Input: part model. Units: mm. Frame: model coordinates. A direction names the side the tool comes from. Give positions to 0.01 mm unless a question says otherwise; leave off trailing zeros. Loops run counter-clockwise (first coordinate to the right, second up) from the corner with the lowest first, then second, coordinate; pieces in that order, holes last. Notation, with made-up numbers: (-31, -10.5) - (-18, -10.5) arc R18 cw to (-18, 7.5) - close; hole circle Ø3 at (72, 38.25). An arc over 180 degrees is marked (long way). Answer as a JSON object with one key per item and string values.
from build123d import *

# Parameters (mm, degrees)
BOSS_EXTRUDE1_DEPTH  = 45.4
LPATTERN1_COUNT      = 2
LPATTERN1_PITCH      = 20
LPATTERN1_COUNT_DIR2 = 2
LPATTERN1_PITCH_DIR2 = 20


with BuildPart() as part:
    # Sketch1 → Boss-Extrude1 (new body)
    with BuildSketch(Plane(origin=(0, 0, 0), x_dir=(0, 0, -1), z_dir=(1, 0, 0))):
        Polygon((19.5, 5.941454138), (19.5, 0), (27, 0), (27, 13), (0, 13), (0, 0), (7.5, 0), (7.5, 5.941454138), align=None)
        with BuildLine():
            Line((7.5, 3.45), (7.5, 2.55))
            ThreePointArc((7.5, 2.55), (7.95, 3), (7.5, 3.45))
        make_face()
        with BuildLine():
            ThreePointArc((19.5, 3.45), (19.05, 3), (19.5, 2.55))
            Line((19.5, 2.55), (19.5, 3.45))
        make_face()
    extrude(amount=BOSS_EXTRUDE1_DEPTH)

    # Sketch3 → M3x0.5 Tapped Hole1 (revolve, cut)
    with BuildSketch(Plane(origin=(12.7, 13, -23.5), x_dir=(0, 0, 1), z_dir=(1, 0, 0))):
        Polygon((0, 0), (0, 4.251075774), (1.25, 3.5), (1.25, 0), align=None)
    m3x0_5_tapped_hole1 = revolve(axis=Axis((12.7, 19.35, -23.5), (0, -1, 0)), mode=Mode.SUBTRACT)

    # LPattern1: M3x0.5 Tapped Hole1 2 × 2
    with Locations(*[(i * LPATTERN1_PITCH, 0, j * LPATTERN1_PITCH_DIR2) for i in range(LPATTERN1_COUNT) for j in range(LPATTERN1_COUNT_DIR2) if (i, j) != (0, 0)]):
        add(m3x0_5_tapped_hole1, mode=Mode.SUBTRACT)


solid = part.part
Item 1: Cut plane B-B (x = 28.5). Return loops of the section in (y, z), then the cut area to 3 significant figures.
Geometry check:
{"outline": "(0, -27) - (13, -27) - (13, 0) - (0, 0) - (0, -7.5) - (2.55, -7.5) arc R0.45 ccw to (3.45, -7.5) - (5.94, -7.5) - (5.94, -19.5) - (3.45, -19.5) arc R0.45 ccw to (2.55, -19.5) - (0, -19.5) - close", "area": "280 mm2"}
Item 2: Contact query for flat-ended pins moving along their axis: P1, Ø2, axis at x = 12.7, z = -23.5, coming from the +Y side; P2, Ø3.5, axis at x = 16, z = -14.5, coming from the -Y side. Output: stop coordinate, or through.
Geometry check:
{"P1": "stops at y = 9.35", "P2": "stops at y = 5.94"}
Item 3: Cut plane A-A (y = 3). Return loops of the section in (x, z).
Geometry check:
{"outline": "(0, -27) - (45.4, -27) - (45.4, -19.05) - (0, -19.05) - close; (0, -7.95) - (45.4, -7.95) - (45.4, 0) - (0, 0) - close"}
Item 4: Material intervals for line 1 (Z direction, x = 32.7, y = 10.3); line 2 (X direction, y = 10.7, z = -23.5); line 3 (Z direction, x = 36, y = 2.25), sorted ascending. Write a range as [from, to].
Geometry check:
{"line 1": "z = [-27, -24.75], [-22.25, -4.75], [-2.25, 0]", "line 2": "x = [0, 11.45], [13.95, 31.45], [33.95, 45.4]", "line 3": "z = [-27, -19.5], [-7.5, 0]"}
Item 5: Access query for faces 4 (the face through (22, 0, -23)), 5 (the face through (31.646, 11.274, -22.828)), 6 (the face through (22, 1, -19.5)), 7 (the face through (22.38, 2.99, -7.95)). Directions: +Z, -Z, +X, -X, +Y, -Y. A direction counts if a zero-diameter tool reaches every point of the face in a straight line with its end or side. Return the directions, or none.
Geometry check:
{"face 4": "+Z, -Z, +X, -X, -Y", "face 5": "+Y", "face 6": "+X, -X, -Y", "face 7": "+X, -X"}
Item 6: Cut plane C-C (z = -16.5). Return loops of the section in (x, y).
Geometry check:
{"outline": "(0, 5.94) - (45.4, 5.94) - (45.4, 13) - (0, 13) - close"}
Item 7: Mould query, pull axis Z, two halves, no side actions, for faces 1 (the face through (22, 13, -14)), 2 (the face through (22, 1, -7.5)), 3 (the face through (22, 6, -27)). Classes: released by +Z, released by -Z, zero draft, split by the parting line, or undercut.
Geometry check:
{"face 1": "zero draft", "face 2": "undercut", "face 3": "released by -Z"}
